CAD build for the part. Positions are in the model's coordinates, mm. A direction names the side the tool comes from. Give positions to 0.01 mm unless a question says otherwise; leave off trailing zeros. Loops run counter-clockwise (first coordinate to the right, second up) from the corner with the lowest first, then second, coordinate; pieces in that order, holes last. Notation, with made-up numbers: (42, 63) - (50, 63) arc R12 ccw to (50, 74) - close; hole circle Ø5 at (-4.75, 34). An arc over 180 degrees is marked (long way). Return JSON: item names as keys, results as strings.
Autodesk Inventor part; units mm, degrees
ref_plane "Work Plane1" through (5, 0, 0) normal (1, 0, 0) x (0, 1, 0)
ref_plane "XZ Plane" through (0, 0, 0) normal (0, 1, 0) x (-1, 0, 0)
ref_plane "XY Plane" through (0, 0, 0) normal (0, 0, 1) x (1, 0, 0)
sketch "Sketch1" plane through (0, 0, 0) normal (0, 1, 0) x (-1, 0, 0)
  arc A0 (4.7697, 1.5) -> (4.7697, -1.5) centre (0, 0) ccw
  circle A1 centre (0, 0) radius 5
  dimension "d0" = 10
extrude "Extrusion1" add sketch "Sketch1" along normal blind 58.3
sketch "Sketch2" plane through (0, 0, 0) normal (0, -1, 0) x (1, 0, 0)
  arc A0 (-4.7697, -1.5) -> (-4.7697, 1.5) centre (0, 0) ccw
  line L0 (-3.2, 1.5) -> (-4.7697, 1.5)
  line L1 (-3.2, -1.5) -> (-3.2, 1.5)
  line L2 (-4.7697, -1.5) -> (-3.2, -1.5)
  circle A1 centre (0, 0) radius 5
extrude "Extrusion2" add sketch "Sketch2" along normal blind 3
sketch "Sketch3" plane through (0, 0, 0) normal (0, 0, 1) x (1, 0, 0)
  line L0 (7.5, -1.5) -> (3.5, -1.5)
  line L1 (3.5, -1.5) -> (3.5, -0.56)
  line L2 (3.5, -0.56) -> (7.5, -0.56)
  line L3 (7.5, -0.56) -> (7.5, -1.5)
  line L4 (-4.7697, -3) -> (5, -3)
  line L5 (5, -3) -> (5, 58.3)
  line L6 (0, -15.26) -> (0, 70.56)
  line L7 (5, -3) -> (5, 58.3)
  line L8 (5, 27.65) -> (17.8962, 27.65)
  line L9 (7.5, 56.8) -> (3.5, 56.8)
  line L10 (3.5, 56.8) -> (3.5, 55.86)
  line L11 (3.5, 55.86) -> (7.5, 55.86)
  line L12 (7.5, 55.86) -> (7.5, 56.8)
  point P0 (0, 0)
  point P1 (0, 55.3)
  dimension "d10" = 0.94
  dimension "d11" = 4
  dimension "d12" = 1.5
  dimension "d21" = 1.5
revolve "Revolution1" cut sketch "Sketch3" angle 360 about axis through (0, -10, 0) along (0, 1, 0)
ref_plane "Work Plane1" through (5, 0, 0) normal (1, 0, 0) x (0, 1, 0)
sketch "Sketch6" plane through (5, 0, 0) normal (1, 0, 0) x (0, 1, 0)
  line L0 (6.94, 1.5) -> (13.94, 1.5)
  line L1 (13.94, 1.5) -> (13.94, -1.5)
  line L2 (13.94, -1.5) -> (6.94, -1.5)
  line L3 (6.94, -1.5) -> (6.94, 1.5)
  circle A0 centre (6.94, 0) radius 1.5
  circle A1 centre (13.94, 0) radius 1.5
  line L4 (-0.56, 5) -> (55.86, 5)
  line L5 (-0.56, -5) -> (55.86, -5)
  line L6 (42.36, 1.5) -> (49.36, 1.5)
  line L7 (49.36, 1.5) -> (49.36, -1.5)
  line L8 (49.36, -1.5) -> (42.36, -1.5)
  line L9 (42.36, -1.5) -> (42.36, 1.5)
  circle A2 centre (42.36, 0) radius 1.5
  circle A3 centre (49.36, 0) radius 1.5
  line L10 (-3, 5) -> (-3, -5)
  line L11 (58.3, -5) -> (58.3, 5)
  line L12 (-0.56, -5) -> (-0.56, 5)
  line L13 (55.86, 5) -> (55.86, -5)
  point P0 (0, 0)
  dimension "d26" = 3
  dimension "d22" = 3
  dimension "d23" = 3.5
  dimension "d24" = 7
  dimension "d25" = 7
  dimension "d27" = 3.5
  dimension "d33" = 7.5
  dimension "d34" = 6.5
extrude "Extrusion4" cut sketch "Sketch6" against normal blind 1.8 contours A0 L3 | L0 A1 L2 A0 | L3 A0 | A1 L1 | L1 A1 | A2 L9 | L6 A3 L8 A2 | L9 A2 | A3 L7 | L7 A3
properties part number "AxeVerticalManivelle" material "Stainless Steel"
1. Drop flat-ended pins along their axis: P1, Ø1.3, axis at x = 4, y = 9.5, coming from the -Z side; P2, Ø0.8, axis at x = 4, y = 44.5, coming from the +Z side; P3, Ø1.3, axis at x = 3.5, y = 47.5, coming from the -Z side. Give the stop position or say it passes through.
Values follow:
{"P1": "stops at z = -3.71", "P2": "stops at z = 3.47", "P3": "stops at z = -4.11"}
2. Pull direction Z, two halves, no side cores. Call faces 1 (the face through (4, 10, -1.5)), 2 (the face through (4, 46, -1.5)), 3 (the face through (0, -3, 0)), 4 (the face through (3.233, -1.023, 1.341)): +Z half, -Z half, draft (parallel to the pull), parting line (faces both ways), or undercut.
Values follow:
{"face 1": "undercut", "face 2": "undercut", "face 3": "draft", "face 4": "parting line"}
3. Cut at A-A, the plane y = 45.5. Write the cut outline in (x, z), plus the area to 3 significant figures.
Values follow:
{"outline": "(-4.77, -1.5) arc R5 ccw to (4.77, -1.5) - (3.2, -1.5) - (3.2, 1.5) - (4.77, 1.5) arc R5 ccw to (-4.77, 1.5) arc R5 ccw to start", "area": "73.4 mm²"}
4. Cut at C-C, the plane z = 0.75. Write the cut outline in (x, y), plus the area to 3 significant figures.
Values follow:
{"outline": "(-4.94, -3) - (4.94, -3) - (4.94, -1.5) - (3.42, -1.5) - (3.42, -0.56) - (4.94, -0.56) - (4.94, 5.64) - (3.2, 5.64) - (3.2, 15.24) - (4.94, 15.24) - (4.94, 41.06) - (3.2, 41.06) - (3.2, 50.66) - (4.94, 50.66) - (4.94, 55.86) - (3.42, 55.86) - (3.42, 56.8) - (4.94, 56.8) - (4.94, 58.3) - (-4.94, 58.3) - (-4.94, 56.8) - (-3.42, 56.8) - (-3.42, 55.86) - (-4.94, 55.86) - (-4.94, -0.56) - (-3.42, -0.56) - (-3.42, -1.5) - (-4.94, -1.5) - close", "area": "567 mm²"}
5. Which spindle directions (+Z, -Z, +X, -X, +Y, -Y) get a long thin tool onto all of the face, cutting with end or side? Do faces 5 (the face through (3.3, 55.86, 2.2)), 6 (the face through (0, 58.3, 0)), 7 (the face through (3.2, 10, 0)). Say none if no direction does.
Values follow:
{"face 5": "none", "face 6": "+Z, -Z, +X, -X, +Y", "face 7": "+X"}
6. Cut at D-D, the plane y = 26. Write the cut outline in (x, z).
Values follow:
{"outline": "(-4.77, -1.5) arc R5 ccw (long way) to (-4.77, 1.5) arc R5 ccw to start"}
7. Cut at B-B, the plane x = 2. Write the cut outline in (y, z).
Values follow:
{"outline": "(-3, -4.58) - (-1.5, -4.58) - (-1.5, -2.87) - (-0.56, -2.87) - (-0.56, -4.58) - (55.86, -4.58) - (55.86, -2.87) - (56.8, -2.87) - (56.8, -4.58) - (58.3, -4.58) - (58.3, 4.58) - (56.8, 4.58) - (56.8, 2.87) - (55.86, 2.87) - (55.86, 4.58) - (-0.56, 4.58) - (-0.56, 2.87) - (-1.5, 2.87) - (-1.5, 4.58) - (-3, 4.58) - close"}
8. Drill centre lines: probe 1 along Y at (x, z) = (-3.75, -0.5); probe 2 along X at (y, z) = (22.5, 0.25); probe 3 along X at (y, z) = (46.5, 0). Where is each one in solid material? Low to high.
Values follow:
{"probe 1": "y = -3 to -1.5, -0.56 to 55.86, 56.8 to 58.3", "probe 2": "x = -4.99 to 4.99", "probe 3": "x = -5 to 3.2"}
